The model under review builds one solid part; all positions refer to its coordinate system, in mm. A direction names the side the tool comes from. Round coordinates to 2 decimals unless told otherwise and drop trailing zeros. Loops run counter-clockwise (first coordinate to the right, second up) from the corner with the lowest first, then second, coordinate; pieces in that order, holes last. Notation, with made-up numbers: M -20.5,-25 L 14.5,-25 A32 ccw 14.5,13 Z; hole C -22.75,26.25 d9. An arc over 180 degrees is marked long. One line per question, with ' | ' between items.
from build123d import *

# Parameters (mm, degrees)
SKETCH1_W            = 32
SKETCH1_H            = 28
BOSS_EXTRUDE1_DEPTH  = 8
SKETCH4_W            = 28
SKETCH4_H            = 20
BOSS_EXTRUDE2_DEPTH  = 8
M5_CLEARANCE_HOLE1_D = 5.3


with BuildPart() as part:
    # Sketch1 → Boss-Extrude1 (new body)
    with BuildSketch(Plane(origin=(0, 0, 0), x_dir=(1, 0, 0), z_dir=(0, 1, 0))):
        with Locations((-5.9, 0)):
            Rectangle(SKETCH1_W, SKETCH1_H)
    extrude(amount=BOSS_EXTRUDE1_DEPTH)

    # Sketch3 → Ø12.0 (12) Diameter Hole1 (revolve, cut)
    with BuildSketch(Plane(origin=(0, 8, 0), x_dir=(0, 0, 1), z_dir=(1, 0, 0))):
        Polygon((0, 0), (0, 8), (6.25, 8), (6, 7.75), (6, 0.25), (6.25, 0), align=None)
    revolve(axis=Axis((0, 14.35, 0), (0, -1, 0)), mode=Mode.SUBTRACT)

    # Sketch4 → Boss-Extrude2 (add)
    with BuildSketch(Plane.ZY.offset(21.9)):
        with Locations((0, 10)):
            Rectangle(SKETCH4_W, SKETCH4_H)
    extrude(amount=-BOSS_EXTRUDE2_DEPTH)

    # M5 Clearance Hole1 (through all)
    with Locations(Plane(origin=(-13.9, 0, 0), x_dir=(0, 0, -1), z_dir=(1, 0, 0))):
        with Locations((-9, 15), (9, 15)):
            Hole(M5_CLEARANCE_HOLE1_D / 2)


solid = part.part
1) Add section A-A on z = 9. State the section outline as (x, y) points, then the cut area to 3 significant figures.
Output values:
outline: M -21.9,0 L 10.1,0 L 10.1,8 L -13.9,8 L -13.9,12.35 L -21.9,12.35 Z; M -21.9,17.65 L -13.9,17.65 L -13.9,20 L -21.9,20 Z | area: 310 mm²
2) Machinability: for faces 1 (the flat face through (-7, 8, 0)), 2 (the cylindrical face through (-17.956, 13.388, -11.103)), which of the approach directions +Z, -Z, +X, -X, +Y, -Y give a long, thin tool a straight path to every point of the face, cutting with its end or side? Answer none if there is none.
Output values:
face 1: +Z, -Z, +X, +Y | face 2: +X, -X
3) Add section C-C on y = 13. State the section outline as (x, z) points.
Output values:
outline: M -21.9,-14 L -13.9,-14 L -13.9,-10.74 L -21.9,-10.74 Z; M -21.9,-7.26 L -13.9,-7.26 L -13.9,7.26 L -21.9,7.26 Z; M -21.9,10.74 L -13.9,10.74 L -13.9,14 L -21.9,14 Z
4) Mouldability with a two-part tool opening along Y and no side actions: class faces 3 (the flat face through (-10, 5, -14)), 4 (the flat face through (-10, 0, 0)), 5 (the cylindrical face through (-17.956, 13.388, 6.897)) as +Y half, -Y half, draft (parallel to the pull), parting line (faces both ways), or undercut.
Output values:
face 3: draft | face 4: -Y half | face 5: undercut
5) Add section B-B on y = 2.25. State the section outline as (x, z) points, then the cut area to 3 significant figures.
Output values:
outline: M -21.9,-14 L 10.1,-14 L 10.1,14 L -21.9,14 Z; hole C 0,0 d12 | area: 783 mm²
6) Add section D-D on x = -15. State the section outline as (y, z) points.
Output values:
outline: M 0,-14 L 20,-14 L 20,14 L 0,14 Z; hole C 15,-9 d5.3; hole C 15,9 d5.3
7) Insertion check: P1, Ø9.5, axis at y = 14, z = 6.5, coming from the +X side; P2, Ø6, axis at x = -2.5, z = -7.5, coming from the +Y side. Each pin has a flat end and moves straight along its axis. Give the tip position at first contact, or say it passes through.
Output values:
P1: stops at x = -13.9 | P2: stops at y = 8
8) For line 1 (Y direction, x = -18.25, z = -9); line 2 (X direction, y = 6.5, z = 0); line 3 (Y direction, x = 2.5, z = 10.75), list the stretches that pass through material, from the lowest coordinate up.
Output values:
line 1: y = 0 to 12.35, 17.65 to 20 | line 2: x = -21.9 to -6, 6 to 10.1 | line 3: y = 0 to 8
